```python
from build123d import *

# Parameters (mm, degrees)
F0_R          = 10
F0_R_2        = 8
F1_DEPTH      = 105
F3_R          = 12.5
F4_DEPTH      = 27
F4_DEPTH_BACK = 5


with BuildPart() as f1:
    # F0 (on Top) → F1 (new body)
    with BuildSketch(Plane.XY):
        Circle(F0_R)
        Circle(F0_R_2, mode=Mode.SUBTRACT)
    extrude(amount=F1_DEPTH)

    # F3 (on face) → F4 (join, two sides)
    with BuildSketch(Plane(origin=(0, 0, 0), x_dir=(0, -1, 0), z_dir=(-1, 0, 0))) as f4_sk:
        with BuildLine():
            ThreePointArc((11.172051, 110.266167), (13.642667, 114.5973), (14.5, 119.509288))
            ThreePointArc((14.5, 119.509288), (-4.920183, 133.149002), (-11.160938, 110.252752))
            ThreePointArc((-11.160938, 110.252752), (-6.435198, 106.515512), (-0.598424, 105.021642))
            ThreePointArc((-0.598424, 105.021642), (-0.271382, 105.011828), (0.055797, 105.009396))
            ThreePointArc((0.055797, 105.009396), (6.198754, 106.401068), (11.172051, 110.266167))
        make_face()
        with Locations((0, 119.509288)):
            Circle(F3_R, mode=Mode.SUBTRACT)
        with BuildLine():
            ThreePointArc((-0.598424, 105.021642), (-6.435198, 106.515512), (-11.160938, 110.252752))
            Line((-11.160938, 110.252752), (-9.952081, 104.985648))
            Line((-9.952081, 104.985648), (-0.598424, 105.021642))
        make_face()
        with BuildLine():
            Line((9.969966, 105.047546), (11.172051, 110.266167))
            ThreePointArc((11.172051, 110.266167), (6.198754, 106.401068), (0.055797, 105.009396))
            Line((0.055797, 105.009396), (9.969966, 105.047546))
        make_face()
    extrude(amount=F4_DEPTH)
    extrude(f4_sk.sketch, amount=-F4_DEPTH_BACK)


solid = f1.part
```
Check sheet for the modelled part. Datum: model origin and axes. Units: mm. Round coordinates to 2 decimals unless told otherwise and drop trailing zeros. Order: outer loops, then holes, each group sorted by start corner. A loop starts at its lowest first (then second) coordinate and runs counter-clockwise, first axis right, second up. Notation, with made-up numbers: (31, 46.25) - (71, 46.25) arc R11 ccw to (71, 52.25) - close; hole circle Ø9 at (38, 68.5). An arc over 180 degrees is marked (long way). Write item = value, one per line.
Q1. Section check C-C (z = 50.5). Record the boundary of the cut face in (x, y).
Computed:
outline = circle Ø20 at (0, 0); hole circle Ø16 at (0, 0)
Q2. Thickness scan on line 1 along Z through (x, y) = (-15, 0); line 2 along X through (y, z) = (3.5, 98.5); line 3 along X through (y, z) = (-12.75, 119). Record the ranges inside material, lowest first.
Computed:
line_1 = 105.01 to 107.01, 132.01 to 134.01
line_2 = -9.37 to -7.19, 7.19 to 9.37
line_3 = -27 to 5
Q3. Go/stop test with flat-tipped pins: pin 1 (8 mm diameter, centred on x = -13, z = 112.5, fed in from +Y); pin 2 (10 mm diameter, centred on x = -19, y = -2.5, fed in from -Z); pin 3 (1.5 mm diameter, centred on y = 10, z = 88, fed in from +X); pin 4 (8.5 mm diameter, centred on y = -4.5, z = 123, fed in from +X). Record where each tip stops, or that it passes through.
Computed:
pin_1 = 14.18
pin_2 = 105.01
pin_3 = 3.8
pin_4 = through
Q4. Section check A-A (x = -19). Record the boundary of the cut face in (y, z), and give its area (3 significant figures).
Computed:
outline = (-14.5, 119.51) arc R14.5 ccw to (-11.17, 110.27) - (-9.97, 105.05) - (-0.06, 105.01) arc R14.5 ccw to (0.6, 105.02) - (9.95, 104.99) - (11.16, 110.25) arc R14.5 ccw (long way) to start; hole circle Ø25 at (0, 119.51)
area = 199 mm^2
Q5. Section check B-B (y = -3.25). Record the boundary of the cut face in (x, z), and give its area (3 significant figures).
Computed:
outline = (-27, 105.02) - (5, 105.02) - (5, 107.44) - (-27, 107.44) - close; (-27, 131.58) - (5, 131.58) - (5, 133.64) - (-27, 133.64) - close; (-9.46, 0) - (-7.31, 0) - (-7.31, 105) - (-9.46, 105) - close; (7.31, 0) - (9.46, 0) - (9.46, 105) - (7.31, 105) - close
area = 594 mm^2
Q6. Draft check along X on faces 1 (the face through (-1.73, -7.81, 51.76)), 2 (the face through (-2.17, -9.76, 51.77)), 3 (the face through (5, 0.1, 106.7)), 4 (the face through (-11.224, 10.565, 107.656)). Enter one of: pulls with the +X half, pulls with the -X half, needs draft (parallel to the pull), parting line crosses it, or undercut.
Computed:
face_1 = undercut
face_2 = parting line crosses it
face_3 = pulls with the +X half
face_4 = needs draft
